from build123d import *

# Parameters (mm, degrees)
ESQUISSE1_W        = 28.5
ESQUISSE1_H        = 16.2
ESQUISSE1_R        = 1.65
BOSS_EXTRU_1_DEPTH = 5.05
BOSS_EXTRU_2_DEPTH = 3.5
CONG_1_R           = 0.1
ESQUISSE3_W        = 6.2
ESQUISSE3_H        = 0.5
BOSS_EXTRU_3_DEPTH = 12
BOSS_EXTRU_4_DEPTH = 4


with BuildPart() as part:
    # Esquisse1 → Boss.-Extru.1 (new, symmetric)
    with BuildSketch(Plane.XY):
        Rectangle(ESQUISSE1_W, ESQUISSE1_H)
        with Locations((-10.866713513, -6.176868734)):
            Circle(ESQUISSE1_R, mode=Mode.SUBTRACT)
        with Locations((10.867466751, 6.17729689)):
            Circle(ESQUISSE1_R, mode=Mode.SUBTRACT)
    extrude(amount=BOSS_EXTRU_1_DEPTH, both=True)

    # Esquisse2 → Boss.-Extru.2 (add, symmetric)
    with BuildSketch(Plane.XY):
        with BuildLine():
            Line((2.75, 8.1), (2.75, 9.628523069))
            Line((2.75, 9.628523069), (-24.53, 11.231815184))
            Line((-24.53, 11.231815184), (-24.53, 14.75))
            ThreePointArc((-24.53, 14.75), (-22.18, 17.1), (-19.83, 14.75))
            Line((-19.83, 14.75), (-19.83, 11.456450954))
            Line((-19.83, 11.456450954), (3.25, 10.1))
            Line((3.25, 10.1), (3.25, 8.1))
            Line((3.25, 8.1), (2.75, 8.1))
        make_face()
    extrude(amount=BOSS_EXTRU_2_DEPTH, both=True)

    # Congé1
    cong_1_edges = [part.edges().sort_by_distance(p)[0] for p in [
        (3.25, 10.1, 0),
        (2.75, 9.628523069, 0),
    ]]
    fillet(cong_1_edges, radius=CONG_1_R)

    # Esquisse3 → Boss.-Extru.3 (add)
    with BuildSketch(Plane(origin=(14.25, 0, 0), x_dir=(0, 0, -1), z_dir=(1, 0, 0))):
        with Locations((0, 2.25)):
            Rectangle(ESQUISSE3_W, ESQUISSE3_H)
        with Locations((0, -3.9)):
            Rectangle(ESQUISSE3_W, ESQUISSE3_H)
    extrude(amount=BOSS_EXTRU_3_DEPTH)

    # Esquisse4 → Boss.-Extru.4 (add, symmetric)
    with BuildSketch(Plane.XY):
        Polygon((2.75, -8.1), (2.75, -11.6), (34.75, -11.6), (34.75, -16.6), (1.75, -16.6), (1.75, -8.1), align=None)
    extrude(amount=BOSS_EXTRU_4_DEPTH, both=True)


solid = part.part
Verification items for the finished model (mm, model axes). A direction names the side the tool comes from. Give positions to 0.01 mm unless a question says otherwise; leave off trailing zeros. Write each loop counter-clockwise with the first axis right and the second up, starting at its lowest first coordinate (ties: lowest second). Pieces come first, ordered by that corner, then holes. Notation, with made-up numbers: M 18,44 L 70,44 A19 cw 70,65 Z; hole C 40,23.25 d3. An arc over 180 degrees is marked long. Put each result on its own line as item: value. Start each with the question number.
1. Go/stop test with flat-tipped pins: pin 1 Ø1 at (x, z) = (-2.5, 1.5) entering from +Y; pin 2 Ø1 at (y, z) = (-2.5, -2.5) entering from +X; pin 3 Ø5 at (y, z) = (-3.5, -1.5) entering from +X. Record where each tip stops, or that it passes through.
2. Set-up check for faces 4 (the face through (-10.75, 10.42, 0.05)), 5 (the face through (1.75, -12, 0)), 6 (the face through (20, 2, 0)): record each of +Z, -Z, +X, -X, +Y, -Y from which the full face is reachable in a straight line by a thin tool's end or side.
3. Section check B-B (z = -1.5). Give the number of separate pieces and of enclosed holes in the cut face, and give its area (3 significant figures).
4. Scan lines: line 1 along Y through (x, z) = (15, -3); line 2 along X through (y, z) = (9, 1); line 3 along X through (y, z) = (15, -1.75). Record each from-to range of solid material in increasing order. Write a range as [from, to].
5. Section check C-C (x = 30). Record the cut outline in (y, z).
6. Section check D-D (x = -22.18). Record the cut outline in (y, z), and give its area (3 significant figures).
7. Draft check along Y on faces 1 (the face through (18, -16.6, 0)), 2 (the face through (3.25, 9, 0)), 3 (the face through (2.75, 9, 0)). Enter one of: +Y half, -Y half, draft (parallel to the pull), parting line (faces both ways), or undercut.
8. Section check A-A (y = 7). Record the cut outline in (x, z).
Answer list:
1. pin 1: y = 10.47
1. pin 2: x = 14.25
1. pin 3: x = 26.25
2. face 4: +Z, -Z, -X
2. face 5: +Z, -Z, -X, -Y
2. face 6: +Z, -Z, +X
3. separate pieces: 1
3. enclosed holes: 2
3. area: 663 mm2
4. line 1: [-16.6, -11.6], [-4.15, -3.65], [2, 2.5]
4. line 2: [2.75, 3.25]
4. line 3: [-24.52, -19.84]
5. outline: M -16.6,-4 L -11.6,-4 L -11.6,4 L -16.6,4 Z
6. outline: M 11.09,-3.5 L 17.1,-3.5 L 17.1,3.5 L 11.09,3.5 Z
6. area: 42.0 mm2
7. face 1: -Y half
7. face 2: draft
7. face 3: undercut
8. outline: M -14.25,-5.05 L 9.44,-5.05 L 9.44,5.05 L -14.25,5.05 Z; M 12.3,-5.05 L 14.25,-5.05 L 14.25,5.05 L 12.3,5.05 Z
